```python
from build123d import *

# Parameters (mm, degrees)
SKETCH1_W                   = 31.242
SKETCH1_H                   = 101.6
BOSS_EXTRUDE1_DEPTH         = 5.08
F_1_4_0_25_DIAMETER_HOLE1_D = 6.35
F_1_8_0_1250_DOWEL_HOLE1_D  = 3.175


with BuildPart() as part:
    # Sketch1 → Boss-Extrude1 (new body)
    with BuildSketch(Plane(origin=(0, 0, 0), x_dir=(1, 0, 0), z_dir=(0, 1, 0))):
        with Locations((15.621, 50.8)):
            Rectangle(SKETCH1_W, SKETCH1_H)
    extrude(amount=BOSS_EXTRUDE1_DEPTH)

    # 1/4 (0.25) Diameter Hole1 (through all)
    with Locations(Plane(origin=(0, 0, 0), x_dir=(-1, 0, 0), z_dir=(0, -1, 0))):
        with Locations((-15.621, 69.85), (-15.621, 88.9)):
            Hole(F_1_4_0_25_DIAMETER_HOLE1_D / 2)

    # 1/8 (0.1250) Dowel Hole1 (through all)
    with Locations(Plane(origin=(15.621, 0, -29.5148), x_dir=(0, 0, -1), z_dir=(0, -1, 0))):
        with Locations((0, 0)):
            Hole(F_1_8_0_1250_DOWEL_HOLE1_D / 2)


solid = part.part
```
Check sheet for the modelled part. Datum: model origin and axes. Units: mm. Give positions to 0.01 mm unless a question says otherwise; leave off trailing zeros. Order: outer loops, then holes, each group sorted by start corner. A loop starts at its lowest first (then second) coordinate and runs counter-clockwise, first axis right, second up. Notation, with made-up numbers: M -3,85.25 L 9,85.25 A21 cw 9,122.25 Z; hole C 37,80.25 d4. An arc over 180 degrees is marked long. Answer in a Markdown table with one row per item. Add a question column.
Q1. Thickness scan on L1, parallel to Z at x = 15.5, y = 2.85; L2, parallel to Z at x = 13.5, y = 1.4; L3, parallel to Z at x = 13, y = 0.6. Record the ranges inside material, lowest first.
Q2. Release check for a two-part mould opening along Z. For faces 1 (the flat face through (15, 3, 0)), 2 (the cylindrical face through (16.96, 2.58, -28.66)), 3 (the flat face through (15, 0, -52)) record: released by +Z, released by -Z, zero draft, split by the parting line, or undercut.
Q3. Gauge pin test, flat end, axial feed: pin 1 Ø10 at (x, z) = (20.5, -56.5) entering from -Y. Record the tip position at first contact, or that the pin passes through.
Q4. Sectioned sample at C-C, the plane z = -90. Record the boundary of the cut face in (x, y), and give its area (3 significant figures).
Q5. Sectioned sample at B-B, the plane y = 2.8. Count the separate pieces of the cut face and the enclosed holes in it, and give its area (3 significant figures).
Q6. Sectioned sample at A-A, the plane z = -69.85. Record the boundary of the cut face in (x, y).
Verdict:
| question | item | result |
|---|---|---|
| 1 | L1 | -101.6 to -92.07, -85.73 to -73.02, -66.68 to -31.1, -27.93 to 0 |
| 1 | L2 | -101.6 to -91.26, -86.54 to -72.21, -67.49 to 0 |
| 1 | L3 | -101.6 to -90.69, -87.11 to -71.64, -68.06 to 0 |
| 2 | face 1 | released by +Z |
| 2 | face 2 | undercut |
| 2 | face 3 | zero draft |
| 3 | pin 1 | y = 0 |
| 4 | outline | M 0,0 L 12.64,0 L 12.64,5.08 L 0,5.08 Z; M 18.6,0 L 31.24,0 L 31.24,5.08 L 18.6,5.08 Z |
| 4 | area | 128 mm² |
| 5 | separate pieces | 1 |
| 5 | enclosed holes | 3 |
| 5 | area | 3,100 mm² |
| 6 | outline | M 0,0 L 12.45,0 L 12.45,5.08 L 0,5.08 Z; M 18.8,0 L 31.24,0 L 31.24,5.08 L 18.8,5.08 Z |
